Read the model definition and answer for the solid it produces. Units are mm, in the model's axes. Face numbers are marked on the shaded views. A direction names the side the tool comes from. Give positions to 0.01 mm unless a question says otherwise; leave off trailing zeros. Order: outer loops, then holes, each group sorted by start corner. A loop starts at its lowest first (then second) coordinate and runs counter-clockwise, first axis right, second up. Notation, with made-up numbers: (-2.75, 6.5) -> (8.25, 6.5) arc R27 cw to (8.25, 35.5) -> close; hole circle Ø11 at (68, 6). An arc over 180 degrees is marked (long way). One line per item, written item: value. Start each with the question number.
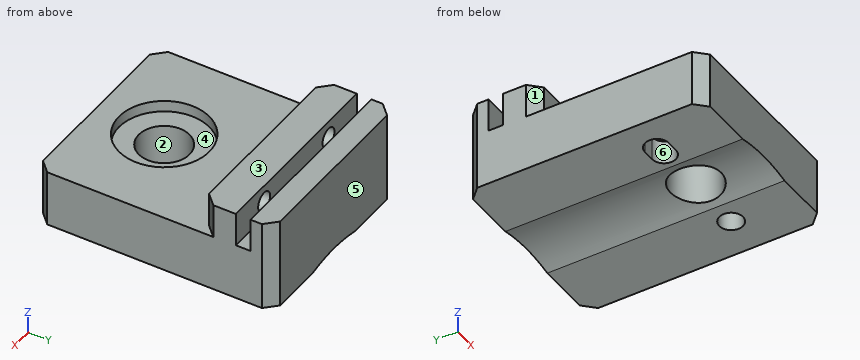
Autodesk Inventor part; units mm, degrees
ref_plane "YZ Plane" through (0, 0, 0) normal (1, 0, 0) x (0, 1, 0)
ref_plane "XZ Plane" through (0, 0, 0) normal (0, 1, 0) x (-1, 0, 0)
ref_plane "XY Plane" through (0, 0, 0) normal (0, 0, 1) x (1, 0, 0)
sketch "Sketch1" plane through (0, 0, 0) normal (0, 0, 1) x (1, 0, 0)
  line L0 (-8.55, 10.5) -> (8.55, 10.5)
  line L1 (8.55, 10.5) -> (8.55, -10.5)
  line L2 (8.55, -10.5) -> (-8.55, -10.5)
  line L3 (-8.55, -10.5) -> (-8.55, 10.5)
  point P0 (0, 0)
  dimension "LENGTH" = 17.1
  dimension "WIDTH" = 21
  dimension "d2" = 10.5
  dimension "d3" = 8.55
extrude "Extrusion1" add sketch "Sketch1" along normal blind 5
sketch "Sketch4" plane through (0, 0, 5) normal (0, 0, 1) x (1, 0, 0)
  line L0 (-8.55, -10.5) -> (8.55, -10.5)
  point P0 (0, 0)
  point P1 (0, -4.5)
  dimension "d16" = 0
  dimension "d17" = 6
hole "Hole1" at (0, -4.5, 5) direction (0, 0, -1) diameter 4.5 depth 5 counterbore diameter 8 counterbore depth 1
sketch "Sketch2" plane through (0, 0, 5) normal (0, 0, 1) x (1, 0, 0)
  line L0 (-8.55, 10.5) -> (8.55, 10.5)
  line L1 (8.55, 10.5) -> (8.55, 4.2)
  line L2 (8.55, 4.2) -> (-8.55, 4.2)
  line L3 (-8.55, 4.2) -> (-8.55, 10.5)
  line L4 (8.55, 6.5) -> (8.55, 5.2)
  line L5 (-8.55, 5.2) -> (-8.55, 6.5)
  point P0 (0, 0)
  dimension "d6" = 10.5
  dimension "d7" = 6.3
  dimension "d8" = 8.55
  dimension "d18" = 17.1
  dimension "d20" = 17.1
extrude "Extrusion2" add sketch "Sketch2" along normal blind 14.05
sketch "Sketch7" plane through (0, 0, 19.05) normal (0, 0, 1) x (1, 0, 0)
  line L0 (8.55, 8.5) -> (-8.55, 8.5)
  line L1 (-8.55, 8.5) -> (-8.55, 7.2)
  line L2 (-8.55, 7.2) -> (8.55, 7.2)
  line L3 (8.55, 7.2) -> (8.55, 8.5)
  line L4 (8.55, 4.2) -> (8.55, 10.5)
  line L5 (-8.55, 4.2) -> (8.55, 4.2)
  line L6 (8.55, 10.5) -> (-8.55, 10.5)
  line L7 (-8.55, 10.5) -> (-8.55, 4.2)
  line L8 (-8.55, 4.2) -> (8.55, 4.2)
  line L9 (8.55, 4.2) -> (8.55, 10.5)
  line L10 (8.55, 10.5) -> (-8.55, 10.5)
  point P0 (0, 0)
  point P1 (-8.55, 4.2)
  point P2 (8.55, 8.5)
  point P3 (8.55, 10.5)
  dimension "d53" = 0
  dimension "d54" = 17.1
  dimension "d55" = 1.3
  dimension "d56" = 3
  dimension "d59" = 0
  dimension "d60" = 0
  dimension "d61" = 0
  dimension "d62" = 0
extrude "Extrusion6" cut sketch "Sketch7" against normal blind 11 contours L0 L7 L6 L4 | L4 L5 L7 L2
extrude "Extrusion5" cut sketch "Sketch7" against normal blind 14 contours L3 L2 L1 L0
sketch "Sketch5" plane through (-8.55, 4.2, 5) normal (0, -1, 0) x (1, 0, 0)
  line L0 (0, 0) -> (0, 3.05)
  line L1 (17.1, 0) -> (17.1, 3.05)
  line L2 (17.1, 3.05) -> (0, 3.05)
  point P0 (8.55, -5)
  point P1 (4, 1.55)
  point P2 (13.1, 1.55)
  point P3 (0, 0.05)
  dimension "d34" = 0
  dimension "d36" = 4
  dimension "d37" = 4
  dimension "d66" = 1.5
hole "Hole2" at (-4.55, 4.2, 6.55) at (4.55, 4.2, 6.55) direction (0, 1, 0) diameter 1.6942 depth 3
sketch "Sketch6" plane through (0, 0, 0) normal (0, 0, -1) x (-1, 0, 0)
  line L0 (5.5, -4.5) -> (4.5, -4.5) construction
  line L1 (5.5, -3.45) -> (4.5, -3.45)
  line L2 (4.5, -5.55) -> (5.5, -5.55)
  arc A0 (5.5, -5.55) -> (5.5, -3.45) centre (5.5, -4.5) ccw
  arc A1 (4.5, -3.45) -> (4.5, -5.55) centre (4.5, -4.5) ccw
  circle A2 centre (0, -4.5) radius 2.25
  point P0 (0, 0)
  point P1 (-5, -4.5)
  point P2 (5, -4.5)
  dimension "d38" = 1
  dimension "d39" = 1.05
  dimension "d40" = 0
  dimension "d41" = 0
  dimension "d42" = 5
  dimension "d43" = 5
hole "Hole3" at (5, -4.5, 0) direction (0, 0, 1) diameter 2.1 depth 2.1
extrude "Extrusion4" cut sketch "Sketch6" against normal blind 2.1 contours A0 L2 A1 L1
chamfer "Chamfer1" distance 1 angle 45 6 edges at (-8.55, 4.2, 6.525) (8.55, 4.2, 6.525) (8.55, 10.5, 4.025) (-8.55, 10.5, 4.025) (8.55, -10.5, 2.5) (-8.55, -10.5, 2.5)
sketch "Sketch8" plane through (-7.55, -10.5, 0) normal (0, -1, 0) x (1, 0, 0)
  circle A0 centre (7.55, -12.35) radius 12.7
  point P0 (7.55, 0)
  dimension "d70" = 0
  dimension "d71" = 12.35
  dimension "d72" = 25.4
extrude "Extrusion7" cut sketch "Sketch8" against normal up to surface (21 mm away)
equation "\"d18\" = LENGTH"
equation "\"d20\" = LENGTH"
equation "\"d23\" = BEAM_HEIGHT - d4"
equation "\"d54\" = LENGTH"
equation "\"d55\" = DICHROIC_THICKNESS + TOLERANCE"
equation "\"TOLERANCE\" = 0.125"
equation "\"BEAM_HEIGHT\" = 19.05"
properties part number "dichroic-mount"
Item 1: Find section C-C on y = 5.75. Write down the section's boundary in (x, z), then the cut area to 3 significant figures.
Item 2: A tool of negligible diameter and unlimited length cuts with its end or side. For the marked faces 4, 5 and 6, from which of +Z, -Z, +X, -X, +Y, -Y can it reach the whole face along a straight path? Write none if from no direction.
Item 3: Flat-ended cylindrical pins translate along their axes: pin 1 (0.9 mm diameter, centred on x = 1, z = 6, fed in from -Y); pin 2 (10 mm diameter, centred on x = -3, y = -4.5, fed in from -Z); pin 3 (9 mm diameter, centred on x = -0.5, y = -2.5, fed in from +Z); pin 4 (5 mm diameter, centred on x = 0, y = -4.5, fed in from -Z). Find the tip coordinate at first contact, or state that the pin passes through.
Item 4: Find section A-A on y = -4.5. Write down the section's boundary in (x, z), then the cut area to 3 significant figures.
Item 5: Find section B-B on x = 0. Write down the section's boundary in (y, z), then the cut area to 3 significant figures.
Item 6: Find the intervals of material crossed by line 1 (X direction, y = -4.5, z = 0.7); line 2 (Y direction, x = 0, z = 2.25); line 3 (Z direction, x = -4.55, y = 6.1), in increasing order. Write a range as from..to.
Item 7: Find section D-D on z = 7. Write down the section's boundary in (x, y), then the cut area to 3 significant figures.
Item 8: For a pull along Y with two mould halves and no side action, classify the marked faces 1, 2 and 3 as +Y half, -Y half, draft (parallel to the pull), parting line (faces both ways), or undercut.
Checks:
1. outline: (-8.55, 0) -> (-2.96, 0) arc R12.7 cw to (2.96, 0) -> (8.55, 0) -> (8.55, 8.05) -> (-8.55, 8.05) -> close; hole circle Ø1.69 at (-4.55, 6.55); hole circle Ø1.69 at (4.55, 6.55)
1. area: 132 mm2
2. face 4: +Z
2. face 5: +Z, -Z, +X, -X, +Y
2. face 6: -Z
3. pin 1: y = 4.2
3. pin 2: z = 0
3. pin 3: z = 5
3. pin 4: z = 0.1
4. outline: (-8.55, 0) -> (-6.55, 0) -> (-6.55, 2.1) -> (-3.45, 2.1) -> (-3.45, 0) -> (-2.96, 0) arc R12.7 cw to (-2.25, 0.15) -> (-2.25, 4) -> (-4, 4) -> (-4, 5) -> (-8.55, 5) -> close; (2.25, 0.15) arc R12.7 cw to (2.96, 0) -> (3.95, 0) -> (3.95, 2.1) -> (6.05, 2.1) -> (6.05, 0) -> (8.55, 0) -> (8.55, 5) -> (4, 5) -> (4, 4) -> (2.25, 4) -> close
4. area: 48.5 mm2
5. outline: (-10.5, 0.35) -> (-6.75, 0.35) -> (-6.75, 4) -> (-8.5, 4) -> (-8.5, 5) -> (-10.5, 5) -> close; (-2.25, 0.35) -> (10.5, 0.35) -> (10.5, 8.05) -> (8.5, 8.05) -> (8.5, 5.05) -> (7.2, 5.05) -> (7.2, 8.05) -> (4.2, 8.05) -> (4.2, 5) -> (-0.5, 5) -> (-0.5, 4) -> (-2.25, 4) -> close
5. area: 88.5 mm2
6. line 1: -8.55..-6.55, -3.45..-2.25, 2.25..3.95, 6.05..8.55
6. line 2: -10.5..-6.75, -2.25..10.5
6. line 3: 0..5.7, 7.4..8.05
7. outline: (-8.55, 5.2) -> (-7.55, 4.2) -> (-5.27, 4.2) -> (-5.27, 7.2) -> (-8.55, 7.2) -> close; (-8.55, 8.5) -> (8.55, 8.5) -> (8.55, 9.5) -> (7.55, 10.5) -> (-7.55, 10.5) -> (-8.55, 9.5) -> close; (-3.83, 4.2) -> (3.83, 4.2) -> (3.83, 7.2) -> (-3.83, 7.2) -> close; (5.27, 4.2) -> (7.55, 4.2) -> (8.55, 5.2) -> (8.55, 7.2) -> (5.27, 7.2) -> close
7. area: 74.9 mm2
8. face 1: -Y half
8. face 2: undercut
8. face 3: draft
